from build123d import *

# Parameters (mm, degrees)
SKETCH1_R           = 1
BOSS_EXTRUDE1_DEPTH = 1.75
SKETCH2_R           = 3.798357005
SKETCH2_R_2         = 2.25
CUT_EXTRUDE1_DEPTH  = 2
CUT_EXTRUDE1_TAPER  = 60
SKETCH3_R           = 3.513551011
SKETCH3_R_2         = 2.25
CUT_EXTRUDE2_DEPTH  = 2
CUT_EXTRUDE2_TAPER  = 60
SCALE1_SCALE        = 18


with BuildPart() as part:
    # Sketch1 → Boss-Extrude1 (new body)
    with BuildSketch(Plane.XY):
        Polygon((2.25, 1.299038106), (0, 2.598076211), (-2.25, 1.299038106), (-2.25, -1.299038106), (0, -2.598076211), (2.25, -1.299038106), align=None)
        Circle(SKETCH1_R, mode=Mode.SUBTRACT)
    extrude(amount=BOSS_EXTRUDE1_DEPTH)

    # Sketch2 → Cut-Extrude1 (cut)
    with BuildSketch(Plane.XY.offset(1.75)):
        Circle(SKETCH2_R)
        Circle(SKETCH2_R_2, mode=Mode.SUBTRACT)
    extrude(amount=-CUT_EXTRUDE1_DEPTH, taper=CUT_EXTRUDE1_TAPER, mode=Mode.SUBTRACT)

    # Sketch3 → Cut-Extrude2 (cut)
    with BuildSketch(Plane(origin=(0, 0, 0), x_dir=(-1, 0, 0), z_dir=(0, 0, -1))):
        Circle(SKETCH3_R)
        Circle(SKETCH3_R_2, mode=Mode.SUBTRACT)
    extrude(amount=-CUT_EXTRUDE2_DEPTH, taper=CUT_EXTRUDE2_TAPER, mode=Mode.SUBTRACT)


with BuildPart() as part_1:
    # Scale1: scaled about (0, 0, 0.875)
    add(part.part.scale(SCALE1_SCALE).moved(Location((0, 0, -14.875))))


solid = part_1.part
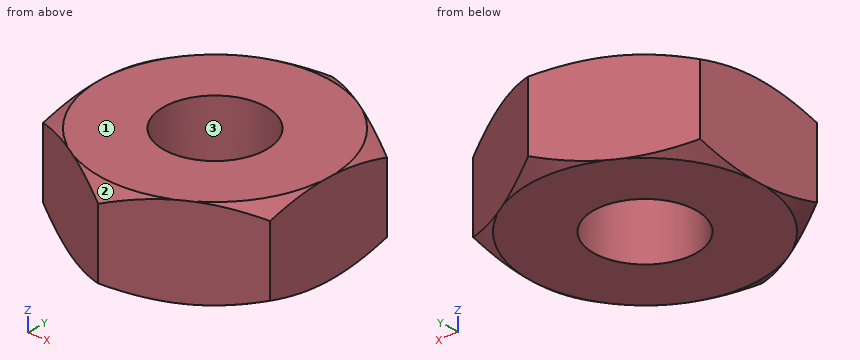
Source: CAD feature listing. Evaluate the final solid. Frame: model axes, mm. Face numbers are marked on the shaded views. Give positions to 0.01 mm unless a question says otherwise; leave off trailing zeros. Loops run counter-clockwise (first coordinate to the right, second up) from the corner with the lowest first, then second, coordinate; pieces in that order, holes last. Notation, with made-up numbers: (75.5, 49.5) -> (103.5, 49.5) arc R22 cw to (103.5, 75.5) -> close; hole circle Ø6 at (29, 62.5). An arc over 180 degrees is marked (long way). Use a Markdown table: item, result. Add a question column.
1) Pull-direction query (X, two-part tool) for the marked faces 1, 2 and 3; classes: +X half, -X half, draft (parallel to the pull), parting line (faces both ways), or undercut.
2) Line query: line 1 along Y through (x, z) = (0, 0); line 2 along Y through (x, z) = (-13.5, 3); line 3 along X through (y, z) = (-41, -5). Output: solid intervals per line, ascending. Write a range as [from, to].
3) First-contact query: pin 1 (1.5 mm diameter, centred on x = -29, z = 5.5, fed in from +Y); pin 2 (8 mm diameter, centred on x = 5, z = -5, fed in from -Y); pin 3 (8 mm diameter, centred on x = 15, z = 11.5, fed in from -Y). Flat tips, straight axial feed; report the tip coordinate or a pass-through.
4) Section query A-A, the plane z = 4. Return the cut outline in (x, y), then the cut area to 3 significant figures.
Numbers:
| question | item | result |
|---|---|---|
| 1 | face 1 | draft |
| 1 | face 2 | parting line |
| 1 | face 3 | undercut |
| 2 | line 1 | y = [-46.77, -18], [18, 46.77] |
| 2 | line 2 | y = [-38.97, -11.91], [11.91, 38.97] |
| 2 | line 3 | x = [-9.99, 9.99] |
| 3 | pin 1 | stops at y = 30.46 |
| 3 | pin 2 | stops at y = -46.19 |
| 3 | pin 3 | stops at y = -40.41 |
| 4 | outline | (-40.5, -23.38) -> (0, -46.77) -> (40.5, -23.38) -> (40.5, 23.38) -> (0, 46.77) -> (-40.5, 23.38) -> close; hole circle Ø36 at (0, 0) |
| 4 | area | 4,660 mm2 |
